Study the drawing (mm; zero at the part's minimum x, y, z) and answer. A direction names the side the tool comes from. Round coordinates to 2 decimals unless told otherwise and drop trailing zeros. Write each loop counter-clockwise with the first axis right and the second up, starting at its lowest first coordinate (ties: lowest second). Pieces come first, ordered by that corner, then holes. Notation, with made-up numbers: (55, 68.5) - (87, 68.5) arc R19 ccw to (87, 79.5) - close; hole circle Ø5 at (-19.5, 59.25). An arc over 180 degrees is marked (long way). Use one line per item in the form item = value. Start each with the question number.
1) The part is cut by section A-A, the plane x = 5. Give the vertices of the cut face in (y, z).
2) The part is cut by section C-C, the plane z = 16.5. Give the vertices of the cut face in (x, y).
3) Each of these flat-tipped pins is pushed along its axis until it touches: pin 1 (1 mm diameter, centred on x = 2.5, z = 4, fed in from -Y); pin 2 (5 mm diameter, centred on x = 5, y = 5, fed in from +Z); pin 3 (8 mm diameter, centred on y = 8.5, z = 8.5, fed in from +X). Where does it stop, or does it pass through?
4) Consider line 1 along Z through (x, y) = (5.25, 4.75); line 2 along Z through (x, y) = (1.75, 7.25); line 3 along X through (y, z) = (2.25, 1) (1 decimal). Determine where each line is inside the solid, lowest interval first. Write a range as from..to.
5) The part is cut by section D-D, the plane x = 3.75. Give the vertices of the cut face in (y, z) (1 decimal).
6) For a pull along X with two mould halves and no side action, classify the marked faces 1, 2, 3 and 4 as released by +X, released by -X, zero draft, split by the parting line, or undercut.
7) The part is cut by section B-B, the plane y = 5. Give the vertices of the cut face in (x, z).
8) For the marked faces 5, 6, 7 and 8, determine the directions among +Z, -Z, +X, -X, +Y, -Y from which every point of the face is accessible in a straight line to the end or side of a thin tool.
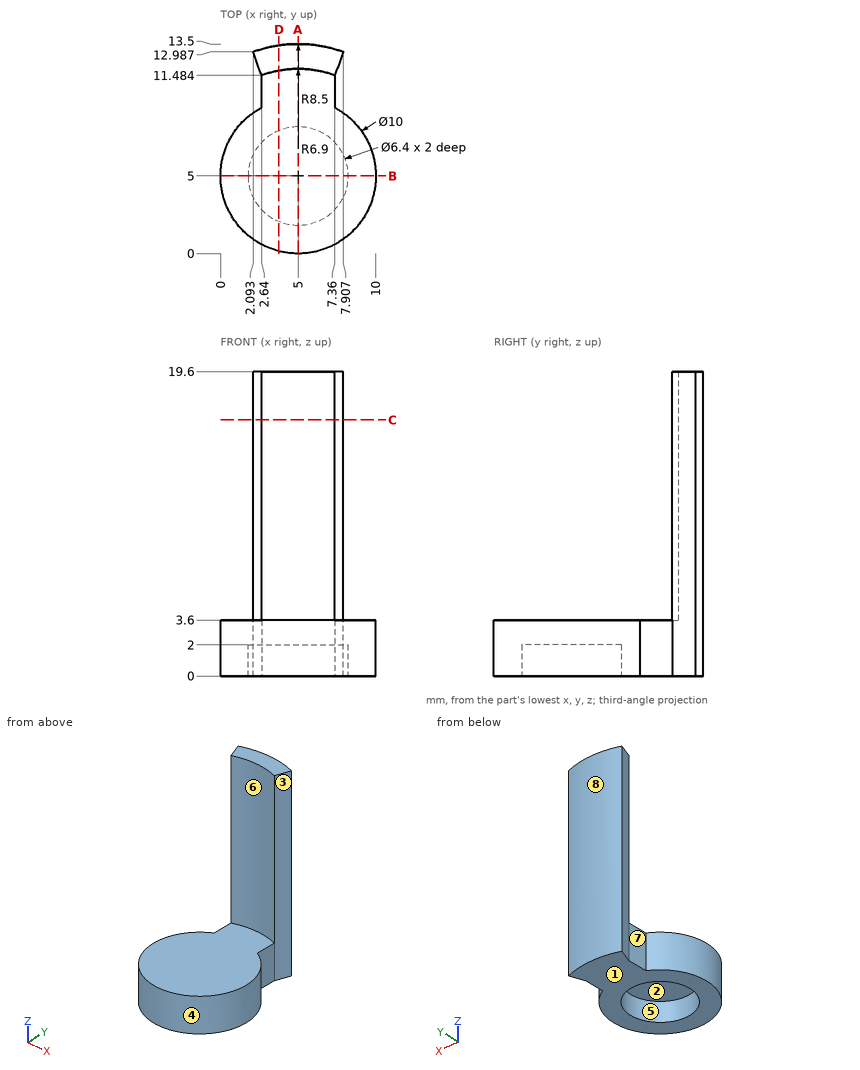
Geometry results:
q1.outline = (0, 0) - (1.8, 0) - (1.8, 2) - (8.2, 2) - (8.2, 0) - (13.5, 0) - (13.5, 19.6) - (11.9, 19.6) - (11.9, 3.6) - (0, 3.6) - close
q2.outline = (2.09, 12.99) - (2.64, 11.48) arc R6.9 cw to (7.36, 11.48) - (7.91, 12.99) arc R8.5 ccw to start
q3.pin_1 = 0.51
q3.pin_2 = 3.6
q3.pin_3 = 7.73
q4.line_1 = 2..3.6
q4.line_2 = 0..3.6
q4.line_3 = 0.8..3.4, 6.6..9.2
q5.outline = (0.2, 0) - (2.1, 0) - (2.1, 2) - (7.9, 2) - (7.9, 0) - (13.4, 0) - (13.4, 19.6) - (11.8, 19.6) - (11.8, 3.6) - (0.2, 3.6) - close
q6.face_1 = zero draft
q6.face_2 = undercut
q6.face_3 = released by +X
q6.face_4 = split by the parting line
q7.outline = (0, 0) - (1.8, 0) - (1.8, 2) - (8.2, 2) - (8.2, 0) - (10, 0) - (10, 3.6) - (0, 3.6) - close
q8.face_5 = -Z
q8.face_6 = +Z, -Y
q8.face_7 = +Z, -Z, -X
q8.face_8 = +Z, -Z, +Y
